Build history of the part. All positions in model axes, mm. A direction names the side the tool comes from. Round coordinates to 2 decimals unless told otherwise and drop trailing zeros. Write each loop counter-clockwise with the first axis right and the second up, starting at its lowest first coordinate (ties: lowest second). Pieces come first, ordered by that corner, then holes. Notation, with made-up numbers: (1.25, -4.75) -> (31.25, -4.75) arc R30 ccw to (31.25, 25.25) -> close; hole circle Ø10 at (84.5, 19.25). An arc over 180 degrees is marked (long way). One line per question, with ' | ' between items.
from build123d import *

# Parameters (mm, degrees)
F1_DEPTH = 3
F2_R     = 1
F4_DEPTH = 1.5


with BuildPart() as f1:
    # F0 (on Top) → F1 (new body)
    with BuildSketch(Plane.XY):
        with BuildLine():
            ThreePointArc((0.75, 7.2), (-10.5, 7.75), (-21.75, 7.2))
            Line((-21.75, 7.2), (-21.75, -0.2))
            ThreePointArc((-21.75, -0.2), (-10.5, -0.75), (0.75, -0.2))
            Line((0.75, -0.2), (0.75, 7.2))
        make_face()
    extrude(amount=F1_DEPTH)

    # F2
    f2_edges = [f1.edges().sort_by_distance(p)[0] for p in [
        (-21.75, 7.2, 1.5),
        (-21.75, -0.2, 1.5),
        (0.75, -0.2, 1.5),
        (0.75, 7.2, 1.5),
    ]]
    fillet(f2_edges, radius=F2_R)

    # F3 (on face) → F4 (join)
    with BuildSketch(Plane.XY.offset(3)):
        with BuildLine():
            Line((2.75, 17.285583), (-23.75, 17.285583))
            Line((-23.75, 17.285583), (-23.75, -0.75))
            ThreePointArc((-23.75, -0.75), (-10.5, -2.75), (2.75, -0.75))
            Line((2.75, -0.75), (2.75, 17.285583))
        make_face()
    extrude(amount=F4_DEPTH)


solid = f1.part
(1) Slice it at C-C (z = 4.05). Write the cut outline in (x, y), then the cut area to 3 significant figures.
Calculated:
outline: (-23.75, -0.75) arc R44.89 ccw to (2.75, -0.75) -> (2.75, 17.29) -> (-23.75, 17.29) -> close | area: 513 mm2
(2) Slice it at A-A (y = 4.25). Write the cut outline in (x, z).
Calculated:
outline: (-23.75, 3) -> (-21.75, 3) -> (-21.75, 0) -> (0.75, 0) -> (0.75, 3) -> (2.75, 3) -> (2.75, 4.5) -> (-23.75, 4.5) -> close
(3) Slice it at D-D (y = 11.5). Write the cut outline in (x, z), then the cut area to 4 significant figures.
Calculated:
outline: (-23.75, 3) -> (2.75, 3) -> (2.75, 4.5) -> (-23.75, 4.5) -> close | area: 39.75 mm2
(4) Slice it at B-B (z = 1.8). Write the cut outline in (x, y), then the cut area to 3 significant figures.
Calculated:
outline: (-21.75, 0.71) arc R1 ccw to (-20.84, -0.29) arc R115.33 ccw to (-0.16, -0.29) arc R1 ccw to (0.75, 0.71) -> (0.75, 6.29) arc R1 ccw to (-0.16, 7.29) arc R115.33 ccw to (-20.84, 7.29) arc R1 ccw to (-21.75, 6.29) -> close | area: 182 mm2
(5) 3-axis set-ups, long thin cutter, end or side, ignore diameter. For faces 1 (the cylindrical face through (-21.495, 0.043, 1.521)), 2 (the flat face through (-21.75, 4, 1)), 3 (the cylindrical face through (-21.481, 6.972, 1.521)), 4 (the cylindrical face through (-10.64, -0.75, 1.48)), 5 (the flat face through (0.75, 3, 1)): which of +Z, -Z, +X, -X, +Y, -Y reach the whole face in a straight line?
Calculated:
face 1: -Z, -X, -Y | face 2: -Z, -X, +Y, -Y | face 3: -Z, -X, +Y | face 4: -Z, -Y | face 5: -Z, +X, +Y, -Y
(6) Drop flat-ended pins along their axis: pin 1 (6 mm diameter, centred on x = -5, y = 11, fed in from -Z); pin 2 (0.9 mm diameter, centred on y = 2.5, z = 1.5, fed in from +X). Give the stop position or say it passes through.
Calculated:
pin 1: z = 3 | pin 2: x = 0.75
(7) Wall check: line 1 (Z direction, x = -14.5, y = 11.25); line 2 (X direction, y = 4, z = 1.9); line 3 (Y direction, x = -4.75, z = 3.2). Give the ranges that are in metal, low to high. Write a range as from..to.
Calculated:
line 1: 3..4.5 | line 2: -21.75..0.75 | line 3: -2.38..17.29
